from build123d import *

# Parameters (mm, degrees)
EXTRUDE_1_DEPTH       = 2
EXTRUDE_2_DEPTH       = 8
SKETCH_6_R            = 3.5
SKETCH_6_R_2          = 1.5
EXTRUDE_10_DEPTH      = 8
SKETCH_7_W            = 121.7
SKETCH_7_H            = 68.8
CUT_EXTRUDE_1_DEPTH   = 10
FILLET_1_R            = 250
SKETCH_6_2_R          = 1.5
EXTRUDE_11_DEPTH      = 1.5
CHAMFER_1_SIZE        = 0.6
CHAMFER_1_SIZE2       = 1.648486452
CUT_EXTRUDE_START     = -6
CUT_EXTRUDE_1_2_DEPTH = 6
SKETCH_12_W           = 7.981613131
SKETCH_12_H           = 4.067552846
SKETCH_12_W_2         = 5
SKETCH_12_H_2         = 2.5
SKETCH_12_W_3         = 6.44213445
SKETCH_12_H_3         = 4.018836203
SKETCH_12_W_4         = 6.293487169
SKETCH_12_H_4         = 3.99394378
SKETCH_12_W_5         = 6.35997617
EXTRUDE_12_DEPTH      = 6.5


with BuildPart() as part:
    # 草图1 → 凸台-拉伸1 (new body)
    with BuildSketch(Plane(origin=(0, 0, 0), x_dir=(1, 0, 0), z_dir=(0, 1, 0))):
        with BuildLine():
            Line((6, 0.2), (143.8, 0.2))
            ThreePointArc((143.8, 0.2), (148.184062043, -1.615937957), (150, -6))
            Line((150, -6), (150, -68.8))
            ThreePointArc((150, -68.8), (148.184062043, -73.184062043), (143.8, -75))
            Line((143.8, -75), (6, -75))
            ThreePointArc((6, -75), (1.615937957, -73.184062043), (-0.2, -68.8))
            Line((-0.2, -68.8), (-0.2, -6))
            ThreePointArc((-0.2, -6), (1.615937957, -1.615937957), (6, 0.2))
        make_face()
    extrude(amount=EXTRUDE_1_DEPTH)

    # 草图1<5> → 拉伸-薄壁2 (add)
    with BuildSketch(Plane(origin=(0, 0, 0), x_dir=(1, 0, 0), z_dir=(0, 1, 0))):
        with BuildLine():
            Line((6, 2.2), (143.8, 2.2))
            ThreePointArc((143.8, 2.2), (149.598275606, -0.201724394), (152, -6))
            Line((152, -6), (152, -68.8))
            ThreePointArc((152, -68.8), (149.598275606, -74.598275606), (143.8, -77))
            Line((143.8, -77), (6, -77))
            ThreePointArc((6, -77), (0.201724394, -74.598275606), (-2.2, -68.8))
            Line((-2.2, -68.8), (-2.2, -6))
            ThreePointArc((-2.2, -6), (0.201724394, -0.201724394), (6, 2.2))
        make_face()
        with BuildLine():
            Line((6, 0.2), (143.8, 0.2))
            ThreePointArc((143.8, 0.2), (148.184062043, -1.615937957), (150, -6))
            Line((150, -6), (150, -68.8))
            ThreePointArc((150, -68.8), (148.184062043, -73.184062043), (143.8, -75))
            Line((143.8, -75), (6, -75))
            ThreePointArc((6, -75), (1.615937957, -73.184062043), (-0.2, -68.8))
            Line((-0.2, -68.8), (-0.2, -6))
            ThreePointArc((-0.2, -6), (1.615937957, -1.615937957), (6, 0.2))
        make_face(mode=Mode.SUBTRACT)
    extrude(amount=EXTRUDE_2_DEPTH)

    # 草图6 → 凸台-拉伸10 (add)
    # profile 1 of 4: a face of its own
    with BuildSketch(Plane(origin=(0, 0, 0), x_dir=(1, 0, 0), z_dir=(0, 1, 0))):
        with Locations((15, 3.7)):
            Circle(SKETCH_6_R)
        with Locations(Location((15, 3.7, 0), (0, 0, 90))):
            Circle(SKETCH_6_R_2, mode=Mode.SUBTRACT)
    # profile 2 of 4: a face of its own
    with BuildSketch(Plane(origin=(0, 0, 0), x_dir=(1, 0, 0), z_dir=(0, 1, 0))):
        with Locations((15, -78.5)):
            Circle(SKETCH_6_R)
        with Locations(Location((15, -78.5, 0), (0, 0, 90))):
            Circle(SKETCH_6_R_2, mode=Mode.SUBTRACT)
    # profile 3 of 4: a face of its own
    with BuildSketch(Plane(origin=(0, 0, 0), x_dir=(1, 0, 0), z_dir=(0, 1, 0))):
        with Locations((134.8, 3.7)):
            Circle(SKETCH_6_R)
        with Locations(Location((134.8, 3.7, 0), (0, 0, 90))):
            Circle(SKETCH_6_R_2, mode=Mode.SUBTRACT)
    # profile 4 of 4: a face of its own
    with BuildSketch(Plane(origin=(0, 0, 0), x_dir=(1, 0, 0), z_dir=(0, 1, 0))):
        with Locations((134.8, -78.5)):
            Circle(SKETCH_6_R)
        with Locations(Location((134.8, -78.5, 0), (0, 0, 90))):
            Circle(SKETCH_6_R_2, mode=Mode.SUBTRACT)
    extrude(amount=EXTRUDE_10_DEPTH)

    # 草图7 → Cut-Extrude 1 (cut)
    with BuildSketch(Plane(origin=(0, 0, 0), x_dir=(-1, 0, 0), z_dir=(0, -1, 0))):
        with Locations((-75.85, -37.4)):
            Rectangle(SKETCH_7_W, SKETCH_7_H)
    extrude(amount=-CUT_EXTRUDE_1_DEPTH, mode=Mode.SUBTRACT)

    # 圆角1
    fillet_1_edges = [part.edges().sort_by_distance(p)[0] for p in [
        (18.16227766, 4, 77),
        (11.83772234, 4, 77),
        (137.96227766, 4, 77),
        (131.63772234, 4, 77),
        (131.63772234, 4, -2.2),
        (137.96227766, 4, -2.2),
        (11.83772234, 4, -2.2),
        (18.16227766, 4, -2.2),
    ]]
    fillet(fillet_1_edges, radius=FILLET_1_R)

    # 草图6<2> → 凸台-拉伸11 (add)
    with BuildSketch(Plane(origin=(0, 0, 0), x_dir=(1, 0, 0), z_dir=(0, 1, 0))):
        with Locations(Location((15, 3.7, 0), (0, 0, 90))):
            Circle(SKETCH_6_2_R)
        with Locations(Location((15, -78.5, 0), (0, 0, 90))):
            Circle(SKETCH_6_2_R)
        with Locations(Location((134.8, 3.7, 0), (0, 0, 90))):
            Circle(SKETCH_6_2_R)
        with Locations(Location((134.8, -78.5, 0), (0, 0, 90))):
            Circle(SKETCH_6_2_R)
    extrude(amount=EXTRUDE_11_DEPTH)

    # 倒角1
    chamfer_1_edges = [part.edges().sort_by_distance(p)[0] for p in [
        (136.7, 0, 37.4),
        (75.85, 0, 71.8),
        (15, 0, 37.4),
        (75.85, 0, 3),
        (14.502874151, 0, 81.964515246),
        (74.9, 0, 77),
        (135.297125849, 0, 81.964515246),
        (150.714252509, 0, 73.20830038),
        (135.297125849, 0, -7.164515246),
        (74.9, 0, -2.2),
        (14.502874151, 0, -7.164515246),
        (-0.914252509, 0, 1.59169962),
        (7.988030543, 0, 78.850628869),
        (40.273083878, 0, 78.235796001),
        (141.811969457, 0, 78.850628869),
        (109.526916122, 0, 78.235796001),
        (141.811969457, 0, -4.050628869),
        (109.526916122, 0, -3.435796001),
        (7.988030543, 0, -4.050628869),
        (40.273083878, 0, -3.435796001),
        (-2.2, 0, 37.4),
        (-0.914252509, 0, 73.20830038),
        (152, 0, 37.4),
        (150.714252509, 0, 1.59169962),
    ]]
    chamfer_1_side = [part.faces().sort_by_distance(p)[0] for p in [
        (0.58783664, 0, 72.250617658),
    ]]
    chamfer(chamfer_1_edges, length=CHAMFER_1_SIZE, length2=CHAMFER_1_SIZE2, reference=chamfer_1_side[0])

    # 草图11 → Cut-Extrude 1 2 (cut)
    with BuildSketch(Plane(origin=(0, 8, 0), x_dir=(1, 0, 0), z_dir=(0, 1, 0)).offset(CUT_EXTRUDE_START)):
        with BuildLine():
            Line((143.8, 0.5), (6, 0.5))
            ThreePointArc((6, 0.5), (1.403805922, -1.403805922), (-0.5, -6))
            Line((-0.5, -6), (-0.5, -68.8))
            ThreePointArc((-0.5, -68.8), (1.403805922, -73.396194078), (6, -75.3))
            Line((6, -75.3), (143.8, -75.3))
            ThreePointArc((143.8, -75.3), (148.396194078, -73.396194078), (150.3, -68.8))
            Line((150.3, -68.8), (150.3, -6))
            ThreePointArc((150.3, -6), (148.396194078, -1.403805922), (143.8, 0.5))
        make_face()
        with BuildLine():
            Line((143.8, 0.2), (6, 0.2))
            ThreePointArc((6, 0.2), (1.615937957, -1.615937957), (-0.2, -6))
            Line((-0.2, -6), (-0.2, -68.8))
            ThreePointArc((-0.2, -68.8), (1.615937957, -73.184062043), (6, -75))
            Line((6, -75), (143.8, -75))
            ThreePointArc((143.8, -75), (148.184062043, -73.184062043), (150, -68.8))
            Line((150, -68.8), (150, -6))
            ThreePointArc((150, -6), (148.184062043, -1.615937957), (143.8, 0.2))
        make_face(mode=Mode.SUBTRACT)
    extrude(amount=CUT_EXTRUDE_1_2_DEPTH, mode=Mode.SUBTRACT)

    # 草图12 → 凸台-拉伸12 (add)
    # profile 1 of 4: a face of its own
    with BuildSketch(Plane(origin=(0, 8, 0), x_dir=(1, 0, 0), z_dir=(0, 1, 0))):
        with Locations((15.444728275, 3.558916951)):
            Rectangle(SKETCH_12_W, SKETCH_12_H)
        with Locations((15, 3.7)):
            Rectangle(SKETCH_12_W_2, SKETCH_12_H_2, mode=Mode.SUBTRACT)
    # profile 2 of 4: a face of its own
    with BuildSketch(Plane(origin=(0, 8, 0), x_dir=(1, 0, 0), z_dir=(0, 1, 0))):
        with Locations((134.555490907, 3.789730855)):
            Rectangle(SKETCH_12_W_3, SKETCH_12_H_3)
        with Locations((134.8, 3.7)):
            Rectangle(SKETCH_12_W_2, SKETCH_12_H_2, mode=Mode.SUBTRACT)
    # profile 3 of 4: a face of its own
    with BuildSketch(Plane(origin=(0, 8, 0), x_dir=(1, 0, 0), z_dir=(0, 1, 0))):
        with Locations((134.721799576, -78.476357082)):
            Rectangle(SKETCH_12_W_4, SKETCH_12_H_4)
        with Locations((134.8, -78.5)):
            Rectangle(SKETCH_12_W_2, SKETCH_12_H_2, mode=Mode.SUBTRACT)
    # profile 4 of 4: a face of its own
    with BuildSketch(Plane(origin=(0, 8, 0), x_dir=(1, 0, 0), z_dir=(0, 1, 0))):
        with Locations((15.237842113, -78.476357082)):
            Rectangle(SKETCH_12_W_5, SKETCH_12_H_4)
        with Locations((15, -78.5)):
            Rectangle(SKETCH_12_W_2, SKETCH_12_H_2, mode=Mode.SUBTRACT)
    extrude(amount=-EXTRUDE_12_DEPTH)


solid = part.part
Could you check a few things on this model? Use its own coordinates, in mm. A direction names the side the tool comes from. Coordinates: 2 decimals unless noted, no trailing zeros. Loops run counter-clockwise (first coordinate to the right, second up) from the corner with the lowest first, then second, coordinate; pieces in that order, holes last.
1. I need wall thicknesses on L1, parallel to Z at x = 15, y = 4.5; L2, parallel to X at y = 2.25, z = 54.5; L3, parallel to Z at x = 136, y = 4. Which ranges of each line are inside material? Lowest first, please.
2. Imagine slicing it at B-B (y = 3.75). Give the number of separate pieces and of enclosed holes in the cut face, and give its area (3 significant figures).
3. We'd pull the mould along X, two halves only. Please class faces 4 (the face through (150.44, 0.65, 72.96)), 5 (the face through (39.93, 4.78, 78.27)), 6 (the face through (69, 0, 2)), 7 (the face through (-0.95, 4.78, 1.65)): released by +X, released by -X, zero draft, split by the parting line, or undercut.
4. Imagine slicing it at A-A (z = 58.5). Please give me the cut outline in (x, y).
5. For faces 1 (the face through (109.18, 4.78, 78.2)), 2 (the face through (74, 5, 75.3)), 3 (the face through (-0.57, 0.65, 73.07)), which set-ups out of +Z, -Z, +X, -X, +Y, -Y let a thin tool reach every point of the face, with its end or its side?
6. For P1, Ø8, axis at x = 59.5, z = 9, coming from the +Y side; P2, Ø1.9, axis at x = 77.5, y = 3.5, coming from the +Z side; P3, Ø2, axis at x = 101, y = 3.5, coming from the -Z side; P4, Ø1.3, axis at x = 135, z = 78.5, coming from the +Y side, each with a flat end and sliding along its axis, tell me the tip position at first contact or that it passes through.
Computed values:
1. L1: z = -7.2 to -4.95, -2.45 to -0.5, 75.3 to 77.25, 79.75 to 82
1. L2: x = -2.2 to -0.5, 150.3 to 152
1. L3: z = -6.99 to -4.6, -2.8 to -0.5, 75.3 to 77.6, 79.4 to 81.79
2. separate pieces: 1
2. enclosed holes: 5
2. area: 1,190 mm2
3. face 4: released by +X
3. face 5: undercut
3. face 6: zero draft
3. face 7: released by -X
4. outline: (-2.2, 1.65) - (-1.6, 0) - (14.4, 0) - (15, 1.65) - (15, 2) - (-0.5, 2) - (-0.5, 8) - (-2.2, 8) - close; (136.7, 1.65) - (137.3, 0) - (151.4, 0) - (152, 1.65) - (152, 8) - (150.3, 8) - (150.3, 2) - (136.7, 2) - close
5. face 1: +Z, +Y, -Y
5. face 2: +Y
5. face 3: +Z, -X, -Y
6. P1: passes through
6. P2: stops at z = 77
6. P3: stops at z = -2.8
6. P4: stops at y = 1.5
